CAD build for the part. Positions are in the model's coordinates, mm. Face numbers are marked on the shaded views. A direction names the side the tool comes from. Give positions to 0.01 mm unless a question says otherwise; leave off trailing zeros. Loops run counter-clockwise (first coordinate to the right, second up) from the corner with the lowest first, then second, coordinate; pieces in that order, holes last.
Solid Edge part; units mm, degrees
sketch "Sketch1" plane through (0, 0, 0) normal (0, 0, 1) x (1, 0, 0)
  circle A0 centre (0, 0) radius 16.2
extrude "Protrusion1" add sketch "Sketch1" against normal blind 1.85
sketch "Sketch2" plane through (0, 0, 0) normal (0, 0, 1) x (1, 0, 0)
  circle A0 centre (0, 0) radius 3.6
  circle A1 centre (0, 0) radius 4.1
extrude "ExtrudedProtrusion_2" add sketch "Sketch2" along normal blind 0.6
sketch "Sketch3" plane through (0, 0, -1.85) normal (0, 0, -1) x (1, 0, 0)
  circle A0 centre (0, 0) radius 4.475
extrude "ExtrudedProtrusion_3" add sketch "Sketch3" along normal blind 2.55
sketch "Sketch4" plane through (0, 0, -4.4) normal (0, 0, -1) x (1, 0, 0)
  circle A0 centre (0, 0) radius 2.9
extrude "ExtrudedCutout_1" cut sketch "Sketch4" against normal blind 4.1
sketch "Sketch5" plane through (0, 0, 0) normal (0, 0, 1) x (1, 0, 0)
  circle A0 centre (0, 0) radius 1.925
extrude "Cutout1" cut sketch "Sketch5" against normal through all
sketch "Sketch6" plane through (0, 0, 0) normal (0, 0, 1) x (1, 0, 0)
  circle A0 centre (-10, 0) radius 1.475
  circle A1 centre (10, 0) radius 1.475
extrude "Cutout2" cut sketch "Sketch6" against normal through all
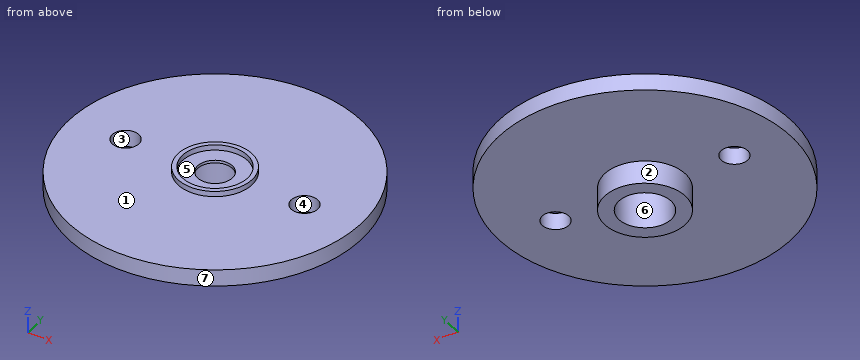
1. Drop flat-ended pins along their axis: pin 1 (7.5 mm diameter, centred on x = 0, y = 0, fed in from -Z); pin 2 (4.5 mm diameter, centred on x = 0, y = 0, fed in from -Z); pin 3 (5 mm diameter, centred on x = -6.5, y = 10.5, fed in from -Z); pin 4 (3.5 mm diameter, centred on x = 0, y = -1, fed in from +Z). Give the stop position or say it passes through.
Responses:
pin 1: stops at z = -4.4
pin 2: stops at z = -0.3
pin 3: stops at z = -1.85
pin 4: stops at z = 0
2. Saw through at D-D, the plane z = -1.45. List the corners of the cut face in (x, y) (3 decimals).
Responses:
outline: circle Ø32.4 at (0, 0); hole circle Ø2.95 at (-10, 0); hole circle Ø5.8 at (0, 0); hole circle Ø2.95 at (10, 0)
3. Saw through at C-C, the plane z = -3.45. List the corners of the cut face in (x, y) (3 decimals).
Responses:
outline: circle Ø8.95 at (0, 0); hole circle Ø5.8 at (0, 0)
4. Pull direction X, two halves, no side cores. Call the marked faces 1, 2, 3 and 4: released by +X, released by -X, zero draft, split by the parting line, or undercut.
Responses:
face 1: zero draft
face 2: split by the parting line
face 3: undercut
face 4: undercut
5. Saw through at A-A, the plane x = 0. List the corners of the cut face in (y, z) (3 decimals).
Responses:
outline: (-16.2, -1.85) - (-4.475, -1.85) - (-4.475, -4.4) - (-2.9, -4.4) - (-2.9, -0.3) - (-1.925, -0.3) - (-1.925, 0) - (-3.6, 0) - (-3.6, 0.6) - (-4.1, 0.6) - (-4.1, 0) - (-16.2, 0) - close; (1.925, -0.3) - (2.9, -0.3) - (2.9, -4.4) - (4.475, -4.4) - (4.475, -1.85) - (16.2, -1.85) - (16.2, 0) - (4.1, 0) - (4.1, 0.6) - (3.6, 0.6) - (3.6, 0) - (1.925, 0) - close
6. Saw through at B-B, the plane y = 0. Count the separate pieces of the cut face and the enclosed holes in it, and give its area (3 significant figures).
Responses:
separate pieces: 4
enclosed holes: 0
area: 47.5 mm2
7. Tool access for the marked faces 5, 6 and 7: list every direction of +Z, -Z, +X, -X, +Y, -Y with a clear straight run to the whole face (end or side of a thin tool).
Responses:
face 5: +Z
face 6: -Z
face 7: +Z, -Z
8. Probe line 1 along Y through (x, z) = (0, -2.65) (3 decimals); line 2 along Y through (x, z) = (0, -1.4); line 3 along Z through (x, y) = (6, -9). List the from-to ranges inside material, lowest first.
Responses:
line 1: y = -4.475 to -2.9, 2.9 to 4.475
line 2: y = -16.2 to -2.9, 2.9 to 16.2
line 3: z = -1.85 to 0
